Input: part model. Units: mm. Frame: model coordinates. A direction names the side the tool comes from. Round coordinates to 2 decimals unless told otherwise and drop trailing zeros. Loops run counter-clockwise (first coordinate to the right, second up) from the corner with the lowest first, then second, coordinate; pieces in that order, holes last. Notation, with made-up numbers: (83, 43) -> (100, 43) arc R16 ccw to (100, 58) -> close; hole circle Ø10 at (-30.5, 3). An arc over 180 degrees is marked (long way). Answer in a Markdown table with one row per item. Add a question column.
Q1. Section A-A, the plane x = 0. Output: boundary loops of the cut face in (y, z).
Q2. Mould query, pull axis X, two halves, no side actions, for faces 6 (the face through (-9.33, -9.45, 4.72)), 7 (the face through (2.889, 8.423, 2.774)), 8 (the face through (9.45, -9.33, 4.72)). Classes: pulls with the +X half, pulls with the -X half, needs draft (parallel to the pull), parting line crosses it, or undercut.
Q3. Reachability of faces 1 (the face through (-8.45, -2.92, 2.77)), 2 (the face through (-4.043, -11.435, 2.726)), 3 (the face through (-3.04, 8.29, 4.7)), 4 (the face through (8.29, 3.04, 4.7)), 5 (the face through (8.45, 2.92, 2.77)) from +Z, -Z, +X, -X, +Y, -Y: full face, straight path, thin tool, end or side. Return the list, or none.
Q4. Section C-C, the plane z = 3.3. Give the number of separate pieces and of enclosed holes in the cut face, and give its area (3 significant figures).
Q5. Ray query, L1, parallel to X at y = -6.5, z = 4.1; L2, parallel to Z at x = 3, y = -6.75; L3, parallel to Y at x = 2.5, z = 2.15. Return the intervals inside material, ascending. Write a range as from..to.
Q6. Pin query (flat end, axial travel): pin 1 (9 mm diameter, centred on x = 0, y = 0, fed in from +Z); pin 2 (1.5 mm diameter, centred on x = -5, y = 7.5, fed in from -Z); pin 3 (2 mm diameter, centred on x = -1, y = -12.5, fed in from +Z); pin 4 (2 mm diameter, centred on x = 8, z = 2, fed in from -Y). Return the tip coordinate at first contact, or that it passes through.
Autodesk Inventor part; units mm, degrees
ref_plane "Work Plane1" through (0, 0, 1) normal (0, 0, 1) x (1, 0, 0)
ref_plane "YZ Plane" through (0, 0, 0) normal (1, 0, 0) x (0, 1, 0)
ref_plane "XZ Plane" through (0, 0, 0) normal (0, 1, 0) x (-1, 0, 0)
sketch "Sketch1" plane through (0, 0, 0) normal (0, 0, 1) x (1, 0, 0)
  circle A0 centre (0, 0) radius 14
  dimension "d0" = 28
extrude "Extrusion1" add sketch "Sketch1" along normal blind 5
chamfer "Chamfer1" distance 1 angle 45 1 edges at (-14, 0, 5)
ref_plane "Work Plane1" through (0, 0, 1) normal (0, 0, 1) x (1, 0, 0)
sketch "Sketch2" plane through (0, 0, 1) normal (0, 0, 1) x (1, 0, 0)
  line L0 (8, 3.25) -> (8, -3.25)
  line L1 (8, 3.25) -> (14.5, 4.75)
  line L2 (14.5, 4.75) -> (14.5, -4.75)
  line L3 (14.5, -4.75) -> (8, -3.25)
  point P0 (0, 0)
  dimension "d7" = 8
  dimension "d8" = 6.5
  dimension "d9" = 3.25
  dimension "d10" = 9.5
  dimension "d11" = 4.75
  dimension "d12" = 6.5
extrude "Extrusion2" cut sketch "Sketch2" along normal blind 5
fillet "Fillet1" radius 2 2 edges at (8, 3.25, 3) (8, -3.25, 3)
chamfer "Chamfer2" distance 0.5 angle 45 5 edges at (10.9197, 3.9238, 5) (8.4348, 2.9041, 5) (8, 0, 5) (8.4348, -2.9041, 5) (10.9197, -3.9238, 5)
pattern_circular "Circular Pattern1" count 4 over 360 about axis through (0, 0, -10) along (0, 0, 1) of "Extrusion2", "Fillet1", "Chamfer2"
sketch "Sketch3" plane through (0, 0, 0) normal (0, 0, -1) x (-1, 0, 0)
  circle A0 centre (0, 0) radius 14
  circle A1 centre (0, 0) radius 12.7
  dimension "d22" = 1.3
extrude "Extrusion3" cut sketch "Sketch3" against normal blind 1 contours A1
sketch "Sketch4" plane through (0, 0, 5) normal (0, 0, 1) x (1, 0, 0)
  arc A0 (-12.1156, -4.7129) -> (-4.7129, -12.1156) centre (0, 0) ccw
hole "Hole1" at (0, 0, 5) direction (0, 0, -1) diameter 11 end through all
chamfer "Chamfer3" distance 0.5 angle 45 1 edges at (0, 5.5, 5)
sketch "Sketch5" plane through (0, 0, 5) normal (0, 0, 1) x (1, 0, 0)
  line L0 (1.659, -7.5) -> (-1.659, -7.5)
  circle A0 centre (0, 0) radius 6
  line L1 (0, 0) -> (-5.6569, 5.6569)
  line L2 (0, 0) -> (-17.4716, 0) construction
  line L3 (0, 0) -> (5.6569, -5.6569) construction
  line L4 (0, 0) -> (6.7175, 6.7175) construction
  line L5 (0, 0) -> (-6.7175, -6.7175) construction
  dimension "d35" = 8
  dimension "d36" = 45
  dimension "d37" = 8
  dimension "d38" = 9.5
  dimension "d39" = 9.5
hole "Hole2" at (-5.6569, 5.6569, 5) at (5.6569, -5.6569, 5) at (-6.7175, -6.7175, 5) at (6.7175, 6.7175, 5) direction (0, 0, -1) diameter 3 end through all
properties part number "base"
Answer block:
| question | item | result |
|---|---|---|
| 1 | outline | (-14, 0) -> (-12.7, 0) -> (-12.7, 1) -> (-14, 1) -> close; (-8, 1) -> (-5.5, 1) -> (-5.5, 4.5) -> (-6, 5) -> (-7.5, 5) -> (-8, 4.5) -> close; (5.5, 1) -> (8, 1) -> (8, 4.5) -> (7.5, 5) -> (6, 5) -> (5.5, 4.5) -> close; (12.7, 0) -> (14, 0) -> (14, 1) -> (12.7, 1) -> close |
| 2 | face 6 | pulls with the -X half |
| 2 | face 7 | undercut |
| 2 | face 8 | pulls with the +X half |
| 3 | face 1 | +Z, -Z, -X |
| 3 | face 2 | +Z, -Y |
| 3 | face 3 | +Z, +Y |
| 3 | face 4 | +Z, +X |
| 3 | face 5 | +Z, -Z, +X |
| 4 | separate pieces | 1 |
| 4 | enclosed holes | 5 |
| 4 | area | 316 mm^2 |
| 5 | L1 | -12.29..-8.2, -5.23..4.42, 6.9..12.29 |
| 5 | L2 | 1..5 |
| 5 | L3 | -8.19..-4.9, 4.9..8.19 |
| 6 | pin 1 | through |
| 6 | pin 2 | z = 1 |
| 6 | pin 3 | z = 1 |
| 6 | pin 4 | y = -12.12 |
